Input: part model. Units: mm. Frame: model coordinates. A direction names the side the tool comes from. Round coordinates to 2 decimals unless told otherwise and drop trailing zeros. Loops run counter-clockwise (first coordinate to the right, second up) from the corner with the lowest first, then second, coordinate; pieces in that order, holes last.
(1) Cut plane D-D, the plane y = 12. Output: boundary loops of the cut face in (x, z), and give its area (3 significant figures).
(2) Access query for faces 4 (the face through (27.31, 61.99, 0.07)), 5 (the face through (20.1, 15, 0)), 6 (the face through (34.674, 53.426, 10.17)). Directions: +Z, -Z, +X, -X, +Y, -Y. A direction counts if a zero-diameter tool reaches every point of the face in a straight line with its end or side. Return the directions, or none.
(3) Cut plane B-B, the plane x = 19. Output: boundary loops of the cut face in (y, z), and give its area (3 significant figures).
(4) First-contact query: pin 1 Ø11 at (x, z) = (6, 0.5) entering from +Y; pin 2 Ø3 at (y, z) = (57.5, 3.5) entering from -X; pin 3 Ø12 at (y, z) = (12, 5) entering from +X; pin 4 Ø6 at (x, z) = (-9.5, 10.5) entering from -Y. Flat tips, straight axial feed; report the tip coordinate or a pass-through.
(5) Line query: line 1 (Z direction, x = 19, y = 28.5); line 2 (X direction, y = 56.5, z = -2); line 3 (Z direction, x = 27.5, y = 15). Output: solid intervals per line, ascending.
(6) Cut plane C-C, the plane y = 22. Output: boundary loops of the cut face in (x, z), and give its area (3 significant figures).
(7) Cut plane A-A, the plane z = -1.75. Output: boundary loops of the cut face in (x, y), and give its area (3 significant figures).
(8) Draft query along Y for faces 1 (the face through (38.94, 45.99, 18.6)), 2 (the face through (37.23, 49, 18.25)), 3 (the face through (0, 15, 3.1)). Return one class per face: released by +Y, released by -Y, zero draft, split by the parting line, or undercut.
from build123d import *

# Parameters (mm, degrees)
BOSS_EXTRUDE1_DEPTH = 30
BOSS_EXTRUDE2_DEPTH = 10.2
CUT_EXTRUDE1_DEPTH  = 10.2
SKETCH4_W           = 15
SKETCH4_H           = 10
BOSS_EXTRUDE3_DEPTH = 2
FILLET1_R           = 5
CUT_EXTRUDE2_REACH  = 85.187
SKETCH5_R           = 3.1


with BuildPart() as part:
    # Sketch1 → Boss-Extrude1 (new body)
    with BuildSketch(Plane(origin=(0, 0, 0), x_dir=(1, 0, 0), z_dir=(0, 1, 0))):
        Polygon((18.1, 3.1), (18.1, 5.1), (22.1, 5.1), (22.1, -5.1), (-22.1, -5.1), (-22.1, 5.1), (-18.1, 5.1), (-20.1, 3.1), (-20.1, -3.1), (20.1, -3.1), (20.1, 3.1), align=None)
    extrude(amount=BOSS_EXTRUDE1_DEPTH)

    # Sketch2 → Boss-Extrude2 (add)
    with BuildSketch(Plane.XY.offset(5.1)):
        Polygon((47.02820323, 34), (29.02820323, 65.176914536), (22.1, 61.176914536), (22.1, 30), (22.1, 0), (40.1, 30), align=None)
    extrude(amount=-BOSS_EXTRUDE2_DEPTH)

    # Sketch3 → Cut-Extrude1 (cut)
    with BuildSketch(Plane.XY.offset(5.1)):
        Polygon((44.346152423, 34.645448267), (28.246152423, 62.531466269), (26.340896534, 61.431466269), (28.140896534, 58.313774815), (24.676794919, 56.313774815), (37.176794919, 34.663139721), (40.640896534, 36.663139721), (42.440896534, 33.545448267), align=None)
    extrude(amount=-CUT_EXTRUDE1_DEPTH, mode=Mode.SUBTRACT)

    # Sketch4 → Boss-Extrude3 (add)
    with BuildSketch(Plane(origin=(49.993584287, 28.863809346, 0), x_dir=(0, 0, -1), z_dir=(0.8660254037844421, 0.49999999999999406, 0))):
        with Locations((-12.6, 23.930762114)):
            Rectangle(SKETCH4_W, SKETCH4_H)
    extrude(amount=-BOSS_EXTRUDE3_DEPTH)

    # Fillet1
    fillet1_edges = [part.edges().sort_by_distance(p)[0] for p in [
        (34.662177826, 53.418584287, 20.1),
        (39.662177826, 44.758330249, 20.1),
    ]]
    fillet(fillet1_edges, radius=FILLET1_R - 0.0001)  # a hair under: the kernel refuses the full size

    # Sketch5 → Cut-Extrude2 (cut, up to next)
    with BuildSketch(Plane(origin=(49.993584287, 28.863809346, 0), x_dir=(0, 0, -1), z_dir=(0.8660254037844421, 0.49999999999999406, 0)), mode=Mode.PRIVATE) as cut_extrude2_sk1:
        with Locations(Location((-15.175304154, 24.225635186, 0), (0, 0, 90))):
            Circle(SKETCH5_R)
    cut_extrude2_tool1 = extrude(cut_extrude2_sk1.sketch, amount=-CUT_EXTRUDE2_REACH, mode=Mode.PRIVATE) & part.part
    add(cut_extrude2_tool1.solids().sort_by_distance((37.880767, 49.843825, 15.175304))[0], mode=Mode.SUBTRACT)


solid = part.part
Reported:
1. outline: (-22.1, -5.1) - (-18.1, -5.1) - (-20.1, -3.1) - (-20.1, 3.1) - (20.1, 3.1) - (20.1, -3.1) - (18.1, -3.1) - (18.1, -5.1) - (29.3, -5.1) - (29.3, 5.1) - (-22.1, 5.1) - close
1. area: 201 mm2
2. face 4: +Z, -Z
2. face 5: +Y, -Y
2. face 6: +Z, -X, +Y
3. outline: (0, -5.1) - (30, -5.1) - (30, -3.1) - (0, -3.1) - close; (0, 3.1) - (30, 3.1) - (30, 5.1) - (0, 5.1) - close
3. area: 120 mm2
4. pin 1: stops at y = 30
4. pin 2: stops at x = 22.1
4. pin 3: stops at x = 32.9
4. pin 4: passes through
5. line 1: z = -5.1 to -3.1, 3.1 to 5.1
5. line 2: x = 22.1 to 25, 31.73 to 34.04
5. line 3: z = -5.1 to 5.1
6. outline: (-22.1, -5.1) - (-18.1, -5.1) - (-20.1, -3.1) - (-20.1, 3.1) - (20.1, 3.1) - (20.1, -3.1) - (18.1, -3.1) - (18.1, -5.1) - (35.3, -5.1) - (35.3, 5.1) - (-22.1, 5.1) - close
6. area: 262 mm2
7. outline: (-22.1, 0) - (-20.1, 0) - (-20.1, 30) - (-22.1, 30) - close; (20.1, 0) - (22.1, 0) - (40.1, 30) - (47.03, 34) - (29.03, 65.18) - (22.1, 61.18) - (22.1, 30) - (20.1, 30) - close; hole (24.68, 56.31) - (37.18, 34.66) - (40.64, 36.66) - (42.44, 33.55) - (44.35, 34.65) - (28.25, 62.53) - (26.34, 61.43) - (28.14, 58.31) - close
7. area: 788 mm2
8. face 1: released by -Y
8. face 2: undercut
8. face 3: zero draft
